Read the model definition and answer for the solid it produces. Units are mm, in the model's axes. A direction names the side the tool comes from. Coordinates: 2 decimals unless noted, no trailing zeros. Order: outer loops, then holes, each group sorted by start corner. A loop starts at its lowest first (then second) coordinate and runs counter-clockwise, first axis right, second up. Notation, with made-up numbers: (45.25, 10.25) -> (104.25, 10.25) arc R28 ccw to (104.25, 41.25) -> close; hole circle Ø9 at (66, 19). An arc over 180 degrees is marked (long way). Use CSV: the item, a comma, the result in double quotes.
Autodesk Inventor part; units mm, degrees
ref_plane "YZ Plane" through (0, 0, 0) normal (1, 0, 0) x (0, 1, 0)
ref_plane "XZ Plane" through (0, 0, 0) normal (0, 1, 0) x (-1, 0, 0)
ref_plane "XY Plane" through (0, 0, 0) normal (0, 0, 1) x (1, 0, 0)
sketch "Sketch1" plane through (0, 0, 0) normal (0, 1, 0) x (-1, 0, 0)
  line L0 (31.1869, 36.5935) -> (-39.9331, 36.5935)
  line L1 (-39.9331, 36.5935) -> (-39.9331, -62.4665)
  line L2 (-39.9331, -62.4665) -> (31.1869, -62.4665)
  line L3 (31.1869, -62.4665) -> (31.1869, 36.5935)
  line L4 (37.5369, 42.9435) -> (-46.2831, 42.9435)
  line L5 (-46.2831, 42.9435) -> (-46.2831, -68.8165)
  line L6 (-46.2831, -68.8165) -> (37.5369, -68.8165)
  line L7 (37.5369, -68.8165) -> (37.5369, 42.9435)
  line L8 (28.6469, 34.0535) -> (-37.3931, 34.0535)
  line L9 (-37.3931, 34.0535) -> (-37.3931, -59.9265)
  line L10 (-37.3931, -59.9265) -> (28.6469, -59.9265)
  line L11 (28.6469, -59.9265) -> (28.6469, 34.0535)
  point P0 (0, 0)
  point P1 (-4.3731, -62.4665)
  point P2 (-4.3731, 36.5935)
  dimension "d0" = 71.12
  dimension "d1" = 99.06
  dimension "d2" = 6.35
  dimension "d3" = 6.35
  dimension "d4" = 6.35
  dimension "d5" = 6.35
  dimension "d22" = 2.54
  dimension "d23" = 2.54
  dimension "d24" = 2.54
  dimension "d25" = 2.54
extrude "Extrusion1" add sketch "Sketch1" against normal blind 44.45 contours L3 L2 L1 L0 | L7 L6 L5 L4 | L11 L10 L9 L8
extrude "Extrusion3" cut sketch "Sketch1" against normal blind 38.1 contours L11 L10 L9 L8
extrude "Extrusion4" cut sketch "Sketch1" against normal blind 24.257 contours L3 L2 L1 L0 | L11 L10 L9 L8
sketch "Sketch5" plane through (-37.5369, 0, 42.9435) normal (0, 0, 1) x (1, 0, 0)
  line L0 (2.54, -2.54) -> (81.28, -2.54)
  line L1 (81.28, -2.54) -> (81.28, -5.588)
  line L2 (81.28, -5.588) -> (2.54, -5.588)
  line L3 (2.54, -5.588) -> (2.54, -2.54)
  line L4 (0, 0) -> (83.82, 0)
  line L5 (83.82, 0) -> (83.82, -44.45)
  line L6 (0, 0) -> (0, -44.45)
  point P0 (37.5369, 0)
  point P1 (81.28, -4.064)
  point P2 (2.54, -4.064)
  dimension "d32" = 2.54
  dimension "d33" = 2.54
  dimension "d34" = 2.54
  dimension "d35" = 3.048
extrude "Extrusion6" cut sketch "Sketch5" against normal blind 108.585
sketch "Sketch6" plane through (39.9331, -24.257, 36.5935) normal (0, 0, -1) x (-1, 0, 0)
  line L0 (71.12, 18.669) -> (71.12, 0)
  line L1 (0, 0) -> (71.12, 0)
  point P0 (39.9331, 24.257)
  point P1 (66.12, 6.35)
  point P2 (56.12, 6.35)
  point P3 (23.12, 6.35)
  point P4 (71.12, 9.3345)
  dimension "d38" = 5
  dimension "d39" = 15
  dimension "d40" = 48
  dimension "d41" = 6.35
  dimension "d42" = 6.35
  dimension "d43" = 6.35
sketch "Sketch7" plane through (37.3931, -38.1, 34.0535) normal (0, 0, -1) x (-1, 0, 0)
  point P0 (37.3931, 38.1)
  point P1 (14.0713, 7.0927)
hole "Hole1" at (-26.1869, -17.907, 36.5935) at (-16.1869, -17.907, 36.5935) at (16.8131, -17.907, 36.5935) direction (0, 0, 1) diameter 6.35 end through all
hole "Hole2" at (23.3218, -31.0073, 34.0535) direction (0, 0, 1) diameter 10.16 end through all
sketch "Sketch8" plane through (-31.1869, -24.257, 36.5935) normal (1, 0, 0) x (0, 0, -1)
  line L0 (0, 18.669) -> (0, 0)
  point P0 (36.5935, 24.257)
  point P1 (60, 8.5086)
  point P2 (0, 9.3345)
  dimension "d58" = 60
hole "Hole3" at (-31.1869, -15.7484, -23.4065) direction (-1, 0, 0) diameter 6.35 end through all
sketch "Sketch9" plane through (46.2831, 0, 42.9435) normal (1, 0, 0) x (0, 0, -1)
  line L0 (0, 0) -> (0, -44.45)
  line L1 (111.76, -44.45) -> (0, -44.45)
  line L2 (0, -41.91) -> (12.7, -41.91)
  line L3 (12.7, -41.91) -> (12.7, -44.45)
  line L4 (12.7, -44.45) -> (0, -44.45)
  line L5 (0, -44.45) -> (0, -41.91)
  line L6 (111.76, -41.91) -> (99.06, -41.91)
  line L7 (99.06, -41.91) -> (99.06, -44.45)
  line L8 (99.06, -44.45) -> (111.76, -44.45)
  line L9 (111.76, -44.45) -> (111.76, -41.91)
  line L10 (111.76, 0) -> (111.76, -44.45)
  point P0 (42.9435, 0)
  point P1 (111.76, -43.18)
  dimension "d66" = 12.7
  dimension "d67" = 12.7
  dimension "d68" = 0
  dimension "d69" = 2.54
  dimension "d70" = 2.54
extrude "Extrusion7" add sketch "Sketch9" along normal blind 12.7
sketch "Sketch10" plane through (46.2831, -41.91, 42.9435) normal (0, 1, 0) x (1, 0, 0)
  point P0 (-46.2831, 42.9435)
  point P1 (6.2127, 6.7401)
  point P2 (6.4208, 105.6569)
hole "Hole4" at (52.4958, -41.91, 36.2034) at (52.7039, -41.91, -62.7134) direction (0, -1, 0) diameter 5.08 end through all
fillet "Fillet1" radius 3.175 2 edges at (46.2831, -41.91, 36.5935) (46.2831, -41.91, -62.4665)
sketch "Sketch11" plane through (-37.5369, 0, -68.8165) normal (-1, 0, 0) x (0, 0, 1)
  line L0 (0, -41.91) -> (12.7, -41.91)
  line L1 (12.7, -41.91) -> (12.7, -44.45)
  line L2 (0, -41.91) -> (12.7, -41.91)
  line L3 (12.7, -41.91) -> (12.7, -44.45)
  line L4 (12.7, -44.45) -> (0, -44.45)
  line L5 (0, -44.45) -> (0, -41.91)
  line L6 (111.76, -41.91) -> (111.76, -44.45)
  line L7 (99.06, -38.735) -> (99.06, -44.45)
  line L8 (111.76, -44.45) -> (99.06, -44.45)
  line L9 (99.06, -44.45) -> (99.06, -41.91)
  line L10 (99.06, -41.91) -> (111.76, -41.91)
  line L11 (111.76, -41.91) -> (111.76, -44.45)
  point P0 (68.8165, 0)
extrude "Extrusion8" add sketch "Sketch11" along normal blind 12.7
sketch "Sketch12" plane through (-37.5369, -41.91, -56.1165) normal (0, 1, 0) x (1, 0, 0)
  point P0 (37.5369, -56.1165)
  point P1 (-6.2476, 6.7674)
  point P2 (-5.9874, -92.7423)
hole "Hole5" at (-43.7845, -41.91, -62.8839) at (-43.5243, -41.91, 36.6258) direction (0, -1, 0) diameter 5.08 end through all
fillet "Fillet2" radius 3.175 2 edges at (-37.5369, -41.91, -62.4665) (-37.5369, -41.91, 36.5935)
properties part number "Housing"
Item 1: Find section C-C, the plane z = 32. Give the vertices of the cut face in (x, y) (3 decimals).
Return value:
outline,"(-50.237, -44.45) -> (58.983, -44.45) -> (58.983, -41.91) -> (49.458, -41.91) arc R3.175 cw to (46.283, -38.735) -> (46.283, 0) -> (39.933, 0) -> (39.933, -2.54) -> (43.743, -2.54) -> (43.743, -5.588) -> (39.933, -5.588) -> (39.933, -24.257) -> (37.393, -24.257) -> (37.393, -38.1) -> (-28.647, -38.1) -> (-28.647, -24.257) -> (-31.187, -24.257) -> (-31.187, -5.588) -> (-34.997, -5.588) -> (-34.997, -2.54) -> (-31.187, -2.54) -> (-31.187, 0) -> (-37.537, 0) -> (-37.537, -38.735) arc R3.175 cw to (-40.712, -41.91) -> (-50.237, -41.91) -> close"
Item 2: The mould has two halves that part along Z. Classify faces 1 (the flat face through (39.933, -1, -12)), 2 (the flat face through (42, -5.588, -3)): +Z half, -Z half, draft (parallel to the pull), parting line (faces both ways), or undercut.
Return value:
face 1,"undercut"
face 2,"draft"
Item 3: Each of these flat-tipped pins is pushed along its axis until it touches: P1, Ø1.5, axis at y = -23.5, z = 5.5, coming from the -X side; P2, Ø20.5, axis at y = -14, z = -31, coming from the +X side; P3, Ø10.5, axis at x = 53, z = -61, coming from the +Y side. Where does it stop, or does it pass through?
Return value:
P1,"stops at x = -37.54"
P2,"stops at x = 46.28"
P3,"stops at y = -41.41"
Item 4: A tool of negligible diameter and unlimited length cuts with its end or side. For faces 3 (the flat face through (-46.5, -41.91, 36.5)), 4 (the flat face through (55.2, -41.91, 36.7)), 5 (the flat face through (37.393, -31, -12)), 6 (the flat face through (-50.237, -43, -63)), 7 (the cylindrical face through (-28.864, -16.2, 39.813)), from which of +Z, -Z, +X, -X, +Y, -Y can it reach the whole face along a straight path? Write none if from no direction.
Return value:
face 3,"+Z, -Z, -X, +Y"
face 4,"+Z, -Z, +X, +Y"
face 5,"+Y"
face 6,"+Z, -Z, -X, +Y, -Y"
face 7,"+Z"
Item 5: Find section A-A, the plane x = 30. Give the vertices of the cut face in (y, z), then the cut area to 3 significant figures.
Return value:
outline,"(-44.45, -68.82) -> (0, -68.82) -> (0, -62.47) -> (-2.54, -62.47) -> (-2.54, -65.64) -> (-5.59, -65.64) -> (-5.59, -62.47) -> (-24.26, -62.47) -> (-24.26, -59.93) -> (-38.1, -59.93) -> (-38.1, 34.05) -> (-24.26, 34.05) -> (-24.26, 36.59) -> (-5.59, 36.59) -> (-5.59, 42.94) -> (-44.45, 42.94) -> close; (-2.54, 36.59) -> (0, 36.59) -> (0, 42.94) -> (-2.54, 42.94) -> close"
area,"1,230 mm^2"
Item 6: Find section D-D, the plane y = -17.5. Give the vertices of the cut face in (x, z).
Return value:
outline,"(-37.54, -68.82) -> (46.28, -68.82) -> (46.28, 42.94) -> (19.96, 42.94) -> (19.96, 36.59) -> (39.93, 36.59) -> (39.93, -62.47) -> (-31.19, -62.47) -> (-31.19, -26.05) -> (-37.54, -26.05) -> close; (-37.54, -20.76) -> (-31.19, -20.76) -> (-31.19, 36.59) -> (-29.34, 36.59) -> (-29.34, 42.94) -> (-37.54, 42.94) -> close; (-23.04, 36.59) -> (-19.34, 36.59) -> (-19.34, 42.94) -> (-23.04, 42.94) -> close; (-13.04, 36.59) -> (13.66, 36.59) -> (13.66, 42.94) -> (-13.04, 42.94) -> close"
Item 7: Straight lines are drawn through the part: line 1 along X through (y, z) = (-30, -9); line 2 along X through (y, z) = (-10, -43.5); line 3 along Z through (x, y) = (-38.5, -43). For each, find the intervals that lie inside material, in ascending order.
Return value:
line 1,"x = -37.54 to -28.65, 37.39 to 46.28"
line 2,"x = -37.54 to -31.19, 39.93 to 46.28"
line 3,"z = -68.82 to -56.12, 30.24 to 42.94"
Item 8: Find section B-B, the plane y = -7. Give the vertices of the cut face in (x, z).
Return value:
outline,"(-37.54, -68.82) -> (46.28, -68.82) -> (46.28, 42.94) -> (-37.54, 42.94) -> close; hole (-31.19, -62.47) -> (39.93, -62.47) -> (39.93, 36.59) -> (-31.19, 36.59) -> close"
